from build123d import *

# Parameters (mm, degrees)
SKETCH1_R           = 8
BOSS_EXTRUDE1_DEPTH = 7
SKETCH2_R           = 1
CUT_EXTRUDE1_DEPTH  = 22


with BuildPart() as part:
    # Sketch1 → Boss-Extrude1 (new body)
    with BuildSketch(Plane.XY):
        with BuildLine():
            Line((-13.5, 8.5), (-8.5, 8.5))
            ThreePointArc((-8.5, 8.5), (-7.155483469, 6.675741758), (-4.941082547, 6.194003868))
            ThreePointArc((-4.941082547, 6.194003868), (0, 7.5), (4.941082547, 6.194003868))
            ThreePointArc((4.941082547, 6.194003868), (7.141563471, 6.697224935), (8.5, 8.5))
            Line((8.5, 8.5), (13.5, 8.5))
            Line((13.5, 8.5), (13.5, -8.5))
            Line((13.5, -8.5), (8, -8.5))
            ThreePointArc((8, -8.5), (0, -12.5), (-8, -8.5))
            Line((-8, -8.5), (-13.5, -8.5))
            Line((-13.5, -8.5), (-13.5, 8.5))
        make_face()
        with Locations((0, -2.5)):
            Circle(SKETCH1_R, mode=Mode.SUBTRACT)
    extrude(amount=BOSS_EXTRUDE1_DEPTH)

    # Sketch2 → Cut-Extrude1 (cut, through all)
    with BuildSketch(Plane(origin=(0, 8.5, 0), x_dir=(1, 0, 0), z_dir=(0, 1, 0))):
        with Locations((-11.5, -3.5)):
            Circle(SKETCH2_R)
        with Locations((11.5, -3.5)):
            Circle(SKETCH2_R)
    extrude(amount=-CUT_EXTRUDE1_DEPTH, mode=Mode.SUBTRACT)


solid = part.part
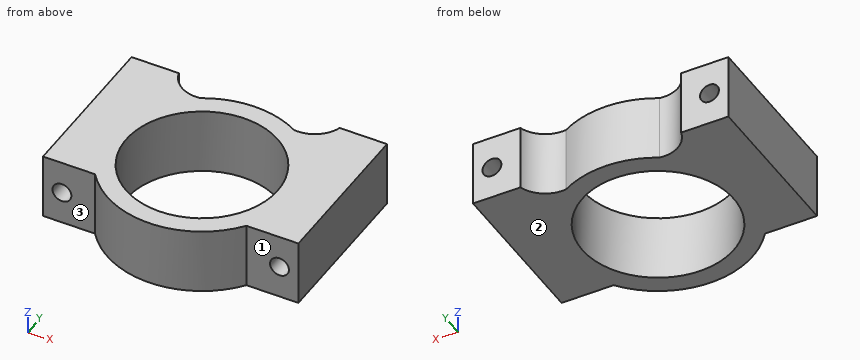
Work out the finished part from the listing and answer in its coordinate system (mm). Face numbers are marked on the shaded views. A direction names the side the tool comes from. Round coordinates to 2 decimals unless told otherwise and drop trailing zeros. Loops run counter-clockwise (first coordinate to the right, second up) from the corner with the lowest first, then second, coordinate; pieces in that order, holes last. Notation, with made-up numbers: (41.25, -38.75) - (98.25, -38.75) arc R10 cw to (98.25, -34.75) - close; hole circle Ø7 at (50, -23). An arc over 180 degrees is marked (long way). Use one line per item in the form item = value. Start each with the question number.
(1) Which of the six approach directions +Z, -Z, +X, -X, +Y, -Y give full straight-line access (tool end or side, diameter ignored) to the marked faces 1, 2 and 3?
(2) Flat-ended cylindrical pins translate along their axes: P1, Ø3, axis at x = 12, z = 2, coming from the -Y side; P2, Ø1.8, axis at x = 11.5, z = 3.5, coming from the +Y side. Find the tip coordinate at first contact, or state that the pin passes through.
(3) Find section A-A on z = 3.5. Determine the outline of the cut face in (x, y).
(4) Find section C-C on x = 0. Determine the outline of the cut face in (y, z).
(5) Find section D-D on z = 5.25. Determine the outline of the cut face in (x, y), and give its area (3 significant figures).
(6) Find section B-B on y = -2.5. Determine the outline of the cut face in (x, z), and give its area (3 significant figures).
(7) Consider line 1 (Z direction, x = -11.5, y = -2); line 2 (X direction, y = 4.5, z = 3.5); line 3 (X direction, y = -2.25, z = 0.75). Determine where each line is inside the solid, lowest interval first.
Answer list:
q1.face_1 = +Z, -Z, +X, -Y
q1.face_2 = -Z, +X, -X, +Y, -Y
q1.face_3 = +Z, -Z, -X, -Y
q2.P1 = -8.5
q2.P2 = through
q3.outline = (-13.5, -8.5) - (-12.5, -8.5) - (-12.5, 8.5) - (-13.5, 8.5) - close; (-10.5, -8.5) - (-8, -8.5) arc R10 ccw to (8, -8.5) - (10.5, -8.5) - (10.5, 8.5) - (8.5, 8.5) arc R3.29 cw to (4.94, 6.19) arc R10 ccw to (-4.94, 6.19) arc R3.21 cw to (-8.5, 8.5) - (-10.5, 8.5) - close; (12.5, -8.5) - (13.5, -8.5) - (13.5, 8.5) - (12.5, 8.5) - close; hole circle Ø16 at (0, -2.5)
q4.outline = (-12.5, 0) - (-10.5, 0) - (-10.5, 7) - (-12.5, 7) - close; (5.5, 0) - (7.5, 0) - (7.5, 7) - (5.5, 7) - close
q5.outline = (-13.5, -8.5) - (-8, -8.5) arc R10 ccw to (8, -8.5) - (13.5, -8.5) - (13.5, 8.5) - (8.5, 8.5) arc R3.29 cw to (4.94, 6.19) arc R10 ccw to (-4.94, 6.19) arc R3.21 cw to (-8.5, 8.5) - (-13.5, 8.5) - close; hole circle Ø16 at (0, -2.5)
q5.area = 276 mm^2
q6.outline = (-13.5, 0) - (-8, 0) - (-8, 7) - (-13.5, 7) - close; (8, 0) - (13.5, 0) - (13.5, 7) - (8, 7) - close; hole circle Ø2 at (-11.5, 3.5); hole circle Ø2 at (11.5, 3.5)
q6.area = 70.7 mm^2
q7.line_1 = 0 to 2.5, 4.5 to 7
q7.line_2 = -13.5 to -12.5, -10.5 to -3.87, 3.87 to 10.5, 12.5 to 13.5
q7.line_3 = -13.5 to -8, 8 to 13.5
